```python
from build123d import *

# Parameters (mm, degrees)
BOSS_EXTRUDE1_DEPTH      = 38
SKETCH2_W                = 26
SKETCH2_H                = 26
CUT_EXTRUDE1_DEPTH       = 178
BOSS_EXTRUDE2_DEPTH      = 26
CHAMFER2_SIZE            = 5
FILLET4_R                = 5
SKETCH4_R                = 19
CUT_EXTRUDE2_DEPTH       = 26
CHAMFER3_SIZE            = 5
CHAMFER3_OF_MIRROR1_SIZE = 5
CHAMFER4_SIZE            = 5
FILLET5_R                = 5


with BuildPart() as part:
    # Sketch1 → Boss-Extrude1 (new, symmetric)
    with BuildSketch(Plane.XY):
        Polygon((0, 139), (0, 0), (127, 0), (127, 50), (38, 139), align=None)
    extrude(amount=BOSS_EXTRUDE1_DEPTH, both=True)

    # Sketch2 → Cut-Extrude1 (cut, along a direction that is not the sketch's normal)
    with BuildSketch(Plane(origin=(0, 139, 0), x_dir=(1, 0, 0), z_dir=(0, 1, 0))):
        with Locations((25, 0)):
            Rectangle(SKETCH2_W, SKETCH2_H)
    extrude(amount=-CUT_EXTRUDE1_DEPTH, dir=(-0.7071067811865489, 0.7071067811865462, 0), mode=Mode.SUBTRACT)

    # Sketch3 → Boss-Extrude2 (add)
    with BuildSketch(Plane.XZ):
        with BuildLine():
            Line((5, 38), (5, 89))
            ThreePointArc((5, 89), (43, 127), (81, 89))
            Line((81, 89), (81, 38))
            Line((81, 38), (5, 38))
        make_face()
    boss_extrude2 = extrude(amount=-BOSS_EXTRUDE2_DEPTH)

    # Chamfer2
    chamfer2_edges = [part.edges().sort_by_distance(p)[0] for p in [
        (5, 26, 63.5),
        (43, 26, 127),
        (81, 26, 63.5),
        (81, 0, 63.5),
        (43, 0, 127),
        (5, 0, 63.5),
    ]]
    chamfer(chamfer2_edges, length=CHAMFER2_SIZE)

    # Fillet4
    fillet4_edges = [part.edges().sort_by_distance(p)[0] for p in [
        (5, 13, 38),
        (81, 13, 38),
        (43, 26, 38),
        (7.5, 2.5, 38),
        (78.5, 2.5, 38),
        (7.5, 23.5, 38),
        (78.5, 23.5, 38),
    ]]
    fillet(fillet4_edges, radius=FILLET4_R - 0.0001)  # a hair under: the kernel refuses the full size

    # Sketch4 → Cut-Extrude2 (cut)
    with BuildSketch(Plane(origin=(0, 26, 0), x_dir=(1, 0, 0), z_dir=(0, 1, 0))):
        with Locations(Location((43, -89, 0), (0, 0, 270))):
            Circle(SKETCH4_R)
    cut_extrude2 = extrude(amount=-CUT_EXTRUDE2_DEPTH, mode=Mode.SUBTRACT)

    # Chamfer3
    chamfer3_edges = [part.edges().sort_by_distance(p)[0] for p in [
        (43, 26, 70),
    ]]
    chamfer(chamfer3_edges, length=CHAMFER3_SIZE)

    # Mirror1: Boss-Extrude2, Cut-Extrude2 across plane
    add(boss_extrude2.mirror(Plane.XY))
    add(cut_extrude2.mirror(Plane.XY), mode=Mode.SUBTRACT)

    # Chamfer3 of Mirror1
    chamfer3_of_mirror1_edges = [part.edges().sort_by_distance(p)[0] for p in [
        (43, 26, -70),
    ]]
    chamfer(chamfer3_of_mirror1_edges, length=CHAMFER3_OF_MIRROR1_SIZE)

    # Chamfer4
    chamfer4_edges = [part.edges().sort_by_distance(p)[0] for p in [
        (81, 0, -63.5),
        (43, 0, -127),
        (5, 0, -63.5),
        (81, 26, -63.5),
        (43, 26, -127),
        (5, 26, -63.5),
    ]]
    chamfer(chamfer4_edges, length=CHAMFER4_SIZE)

    # Fillet5
    fillet5_edges = [part.edges().sort_by_distance(p)[0] for p in [
        (5, 13, -38),
        (81, 13, -38),
        (43, 26, -38),
        (7.5, 2.5, -38),
        (78.5, 2.5, -38),
        (7.5, 23.5, -38),
        (78.5, 23.5, -38),
    ]]
    fillet(fillet5_edges, radius=FILLET5_R - 0.0001)  # a hair under: the kernel refuses the full size


solid = part.part
```
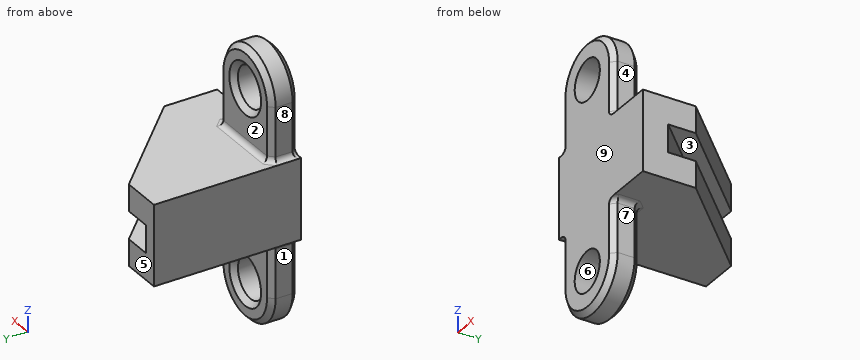
Build history of the part. All positions in model axes, mm. Face numbers are marked on the shaded views. A direction names the side the tool comes from. Coordinates: 2 decimals unless noted, no trailing zeros. Write each loop counter-clockwise with the first axis right and the second up, starting at its lowest first coordinate (ties: lowest second). Pieces come first, ordered by that corner, then holes.
1. 3-axis set-ups, long thin cutter, end or side, ignore diameter. For the marked faces 1, 2, 3, 4 and 5: which of +Z, -Z, +X, -X, +Y, -Y reach the whole face in a straight line?
Answer block:
face 1: -Z, -X, +Y, -Y
face 2: +Z, +X, -X, +Y
face 3: +X, +Y
face 4: +Z, +X, +Y, -Y
face 5: +Z, -Z, +X, -X, +Y
2. Drill centre lines: probe 1 along Z at (x, y) = (83, 89.5); probe 2 along Z at (x, y) = (92, 58); probe 3 along Z at (x, y) = (25.5, 13.5). Where is each one in solid material? Low to high.
Answer block:
probe 1: z = -38 to -13, 13 to 38
probe 2: z = -38 to 38
probe 3: z = -122.73 to -96.4, -81.6 to 81.6, 96.4 to 122.73
3. Band-saw the part on C-C, the plane z = 21.5. Give the cut face in (x, y), and give its area (3 significant figures).
Answer block:
outline: (0, 0) - (127, 0) - (127, 50) - (38, 139) - (0, 139) - close
area: 13,700 mm2
4. Band-saw the part on D-D, the plane y = 97. Give the cut face in (x, z), and give its area (3 significant figures).
Answer block:
outline: (0, -38) - (80, -38) - (80, -13) - (54, -13) - (54, 13) - (80, 13) - (80, 38) - (0, 38) - close
area: 5,400 mm2
5. Band-saw the part on A-A, the plane x = 43. Give the number of separate pieces and of enclosed holes in the cut face, and give its area (3 significant figures).
Answer block:
separate pieces: 3
enclosed holes: 0
area: 12,100 mm2
6. Drop flat-ended pins along their axis: pin 1 (8 mm diameter, centred on y = 16, z = 58.5, fed in from -X); pin 2 (6 mm diameter, centred on x = 77.5, z = -31, fed in from +Y); pin 3 (17.5 mm diameter, centred on y = 13, z = -59.5, fed in from +X). Give the stop position or say it passes through.
Answer block:
pin 1: stops at x = 5
pin 2: stops at y = 102.5
pin 3: stops at x = 81
7. Pull direction X, two halves, no side cores. Call the marked faces 6, 7, 8 and 9: released by +X, released by -X, zero draft, split by the parting line, or undercut.
Answer block:
face 6: undercut
face 7: released by +X
face 8: released by -X
face 9: zero draft
